Model file for the job. Use its own axes, mm. Round coordinates to 2 decimals unless told otherwise and drop trailing zeros. Loops run counter-clockwise (first coordinate to the right, second up) from the corner with the lowest first, then second, coordinate; pieces in that order, holes last.
from build123d import *

# Parameters (mm, degrees)
SKETCH1_R           = 1.4732
BOSS_EXTRUDE1_DEPTH = 5.08
SKETCH2_R           = 71.5
BOSS_EXTRUDE2_DEPTH = 5.08


with BuildPart() as part:
    # Sketch1 → Boss-Extrude1 (new body)
    with BuildSketch(Plane(origin=(0, 0, 0), x_dir=(0, 0, -1), z_dir=(1, 0, 0))):
        with BuildLine():
            Line((-134.851685393, 37.21011236), (114.148314607, 37.21011236))
            ThreePointArc((114.148314607, 37.21011236), (139.148314607, 12.21011236), (114.148314607, -12.78988764))
            Line((114.148314607, -12.78988764), (-134.851685393, -12.78988764))
            ThreePointArc((-134.851685393, -12.78988764), (-159.851685393, 12.21011236), (-134.851685393, 37.21011236))
        make_face()
        with Locations((-134.851685393, 12.21011236)):
            Circle(SKETCH1_R, mode=Mode.SUBTRACT)
        with Locations((114.148314607, 12.21011236)):
            Circle(SKETCH1_R, mode=Mode.SUBTRACT)
    extrude(amount=BOSS_EXTRUDE1_DEPTH)

    # Sketch2 → Boss-Extrude2 (add)
    with BuildSketch(Plane(origin=(5.08, 0, 0), x_dir=(0, 0, -1), z_dir=(1, 0, 0))):
        with Locations((165.767109633, 63.828907386)):
            Circle(SKETCH2_R)
    extrude(amount=-BOSS_EXTRUDE2_DEPTH)


solid = part.part
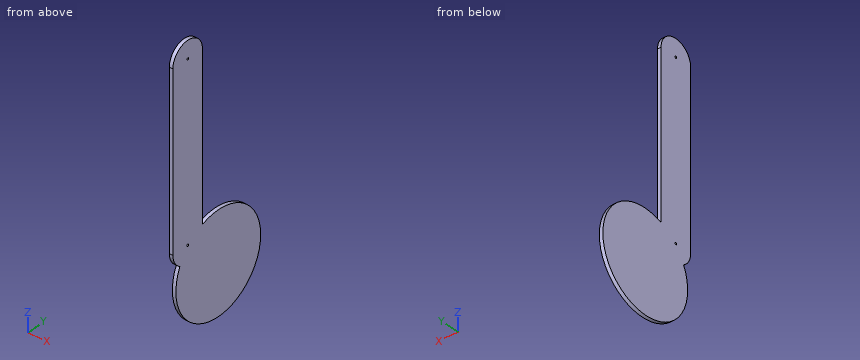
Q1. Slice it at A-A on x = 2. Give the cut face in (y, z), plus the area to 3 significant figures.
Q2. Slice it at C-C on y = 81. Give the cut face in (x, z).
Q3. Flat gauge pins, fed straight in: P1, Ø1.5, axis at x = 1, z = -137.5, coming from the -Y side; P2, Ø2.5, axis at x = 3, z = 60.5, coming from the +Y side; P3, Ø3, axis at x = 1.5, z = -128.5, coming from the +Y side. Where does each tip first touch, or does it go through?
Q4. Slice it at B-B on z = -25.5. Give the cut face in (x, y), plus the area to 3 significant figures.
Q5. Probe line 1 (Z direction, x = 2.7, y = 11); line 2 (Y direction, x = 1.6, z = -35); line 3 (Z direction, x = 2.05, y = 35). List the from-to ranges inside material, lowest first.
Reply:
1. outline: (-12.79, -114.15) arc R25 ccw to (-0.91, -135.43) arc R71.5 ccw (long way) to (37.21, -99.41) - (37.21, 134.85) arc R25 ccw to (-12.79, 134.85) - close; hole circle Ø2.95 at (12.21, -114.15); hole circle Ø2.95 at (12.21, 134.85)
1. area: 29,600 mm2
2. outline: (0, -235.17) - (5.08, -235.17) - (5.08, -96.36) - (0, -96.36) - close
3. P1: stops at y = -2.16
3. P2: stops at y = 37.21
3. P3: stops at y = 125.74
4. outline: (0, -12.79) - (5.08, -12.79) - (5.08, 37.21) - (0, 37.21) - close
4. area: 254 mm2
5. line 1: z = -213.95 to -114.99, -113.31 to 134.01, 135.69 to 159.82
5. line 2: y = -12.79 to 37.21
5. line 3: z = -231.2 to 145.13
